```python
from build123d import *

# Parameters (mm, degrees)
F1_DEPTH = 7
F2_R     = 1.5875


with BuildPart() as f1:
    # F0 (on Top) → F1 (new body)
    with BuildSketch(Plane.XY):
        with BuildLine():
            ThreePointArc((11.0716033166, 9.525), (13.6931879312, 5.0796288526), (14.605, 0))
            Line((14.605, 0), (44.45, 0))
            Line((44.45, 0), (44.45, 9.525))
            Line((44.45, 9.525), (11.0716033166, 9.525))
        make_face()
        with BuildLine():
            Line((44.45, 0), (14.605, 0))
            ThreePointArc((14.605, 0), (13.6931879312, -5.0796288526), (11.0716033166, -9.525))
            Line((11.0716033166, -9.525), (44.45, -9.525))
            Line((44.45, -9.525), (44.45, 0))
        make_face()
        with BuildLine():
            ThreePointArc((-5.5022154629, 9.525), (0, 11), (5.5022154629, 9.525))
            Line((5.5022154629, 9.525), (11.0716033166, 9.525))
            ThreePointArc((11.0716033166, 9.525), (0, 14.605), (-11.0716033166, 9.525))
            Line((-11.0716033166, 9.525), (-5.5022154629, 9.525))
        make_face()
        with BuildLine():
            Line((11.0716033166, -9.525), (5.5022154629, -9.525))
            ThreePointArc((5.5022154629, -9.525), (0, -11), (-5.5022154629, -9.525))
            Line((-5.5022154629, -9.525), (-11.0716033166, -9.525))
            ThreePointArc((-11.0716033166, -9.525), (0, -14.605), (11.0716033166, -9.525))
        make_face()
        with BuildLine():
            Line((-16.9569512222, -9.525), (-11.0716033166, -9.525))
            ThreePointArc((-11.0716033166, -9.525), (-13.6931879312, -5.0796288526), (-14.605, 0))
            Line((-14.605, 0), (-18.21, 0))
            ThreePointArc((-18.21, 0), (-29.21, -11), (-40.21, 0))
            Line((-40.21, 0), (-44.45, 0))
            Line((-44.45, 0), (-44.45, -6.35))
            Line((-44.45, -6.35), (-11.3722009461, -34.1055689863))
            Line((-11.3722009461, -34.1055689863), (-1.5761177745, -22.4310516731))
            Line((-1.5761177745, -22.4310516731), (-16.9569512222, -9.525))
        make_face()
        with BuildLine():
            ThreePointArc((5.5022154629, 9.525), (9.5269189692, 5.498892157), (11, 0))
            Line((11, 0), (14.605, 0))
            ThreePointArc((14.605, 0), (13.6931879312, 5.0796288526), (11.0716033166, 9.525))
            Line((11.0716033166, 9.525), (5.5022154629, 9.525))
        make_face()
        with BuildLine():
            ThreePointArc((-11, 0), (-9.5269189692, 5.498892157), (-5.5022154629, 9.525))
            Line((-5.5022154629, 9.525), (-11.0716033166, 9.525))
            ThreePointArc((-11.0716033166, 9.525), (-13.6931879312, 5.0796288526), (-14.605, 0))
            Line((-14.605, 0), (-11, 0))
        make_face()
        with BuildLine():
            Line((-11.0716033166, -9.525), (-5.5022154629, -9.525))
            ThreePointArc((-5.5022154629, -9.525), (-9.5269189692, -5.498892157), (-11, 0))
            Line((-11, 0), (-14.605, 0))
            ThreePointArc((-14.605, 0), (-13.6931879312, -5.0796288526), (-11.0716033166, -9.525))
        make_face()
        with BuildLine():
            Line((14.605, 0), (11, 0))
            ThreePointArc((11, 0), (9.5269189692, -5.498892157), (5.5022154629, -9.525))
            Line((5.5022154629, -9.525), (11.0716033166, -9.525))
            ThreePointArc((11.0716033166, -9.525), (13.6931879312, -5.0796288526), (14.605, 0))
        make_face()
        with BuildLine():
            ThreePointArc((-14.605, 0), (-13.6931879312, 5.0796288526), (-11.0716033166, 9.525))
            Line((-11.0716033166, 9.525), (-16.9569512222, 9.525))
            Line((-16.9569512222, 9.525), (-1.5761177745, 22.4310516731))
            Line((-1.5761177745, 22.4310516731), (-11.3722009461, 34.1055689863))
            Line((-11.3722009461, 34.1055689863), (-44.45, 6.35))
            Line((-44.45, 6.35), (-44.45, 0))
            Line((-44.45, 0), (-40.21, 0))
            ThreePointArc((-40.21, 0), (-29.21, 11), (-18.21, 0))
            Line((-18.21, 0), (-14.605, 0))
        make_face()
    extrude(amount=F1_DEPTH)

    # F2
    f2_edges = [f1.edges().sort_by_distance(p)[0] for p in [
        (-44.45, -6.35, 3.5),
        (-11.372201, -34.105569, 3.5),
        (-27.9111, -20.227784, 0),
        (-27.9111, -20.227784, 7),
        (-1.576118, -22.431052, 3.5),
        (-6.474159, -28.26831, 0),
        (-6.474159, -28.26831, 7),
        (44.45, -9.525, 3.5),
        (44.45, 9.525, 3.5),
        (44.45, 0, 0),
        (44.45, 0, 7),
        (-1.576118, 22.431052, 3.5),
        (-11.372201, 34.105569, 3.5),
        (-6.474159, 28.26831, 0),
        (-6.474159, 28.26831, 7),
        (-44.45, 0, 7),
        (-44.45, 6.35, 3.5),
        (-44.45, 0, 0),
        (-27.9111, 20.227784, 0),
        (-27.9111, 20.227784, 7),
        (-9.266534, 15.978026, 7),
        (-14.014277, 9.525, 7),
        (-9.266534, 15.978026, 0),
        (-14.014277, 9.525, 0),
        (0, 14.605, 0),
        (0, 14.605, 7),
        (27.760802, 9.525, 7),
        (27.760802, 9.525, 0),
        (27.760802, -9.525, 7),
        (0, -14.605, 7),
        (-14.014277, -9.525, 7),
        (-9.266534, -15.978026, 7),
        (-9.266534, -15.978026, 0),
        (27.760802, -9.525, 0),
        (0, -14.605, 0),
        (-14.014277, -9.525, 0),
    ]]
    fillet(f2_edges, radius=F2_R)


solid = f1.part
```
For this review, take the finished solid that the model builds, in its own axes (mm). A direction names the side the tool comes from. Round coordinates to 2 decimals unless told otherwise and drop trailing zeros.
Q1. Machinability: for faces 4 (the face through (-9.775, -15.551, 3.473)), 5 (the face through (-10.01, -15.94, 0.48)), 6 (the face through (27, 9.525, 3)), which of the approach directions +Z, -Z, +X, -X, +Y, -Y give a long, thin tool a straight path to every point of the face, cutting with its end or side? Answer none if there is none.
Result sheet:
face 4: +Z, -Z
face 5: -Z
face 6: +Z, -Z, +X, +Y
Q2. To check wall thickness, follow line 1 along Y through (x, z) = (-5.5, 2.25); line 2 along Y through (x, z) = (-15.5, 4.5) (3 decimals); line 3 along X through (y, z) = (-6, 5). State the ranges of each line that lie inside material, in increasing order.
Result sheet:
line 1: y = -27.11 to -19.14, -13.53 to -9.53, 9.53 to 13.53, 19.14 to 27.11
line 2: y = -30.642 to -10.748, -9.525 to 9.525, 10.748 to 30.642
line 3: x = -44.4 to -38.43, -19.99 to -9.22, 9.22 to 44.45
Q3. Insertion check: pin 1 Ø1.5 at (x, z) = (-24, 2) entering from +Y; pin 2 Ø1.1 at (x, z) = (23.5, 3.5) entering from -Y (3 decimals); pin 3 Ø3 at (x, z) = (27, 3.5) entering from +Y (3 decimals). Each pin has a flat end and moves straight along its axis. Give the tip position at first contact, or say it passes through.
Result sheet:
pin 1: stops at y = 24.14
pin 2: stops at y = -9.525
pin 3: stops at y = 9.525
Q4. Add section A-A on y = 0. Give the number of separate pieces and of enclosed holes in the cut face, plus the area to 3 significant figures.
Result sheet:
separate pieces: 3
enclosed holes: 0
area: 312 mm2
Q5. Mouldability with a two-part tool opening along X and no side actions: class faces 1 (the face through (-10.01, -15.94, 6.52)), 2 (the face through (-7, -9, 7)), 3 (the face through (-6.767, -27.913, 6.523)) as +X half, -X half, draft (parallel to the pull), parting line (faces both ways), or undercut.
Result sheet:
face 1: undercut
face 2: draft
face 3: +X half
